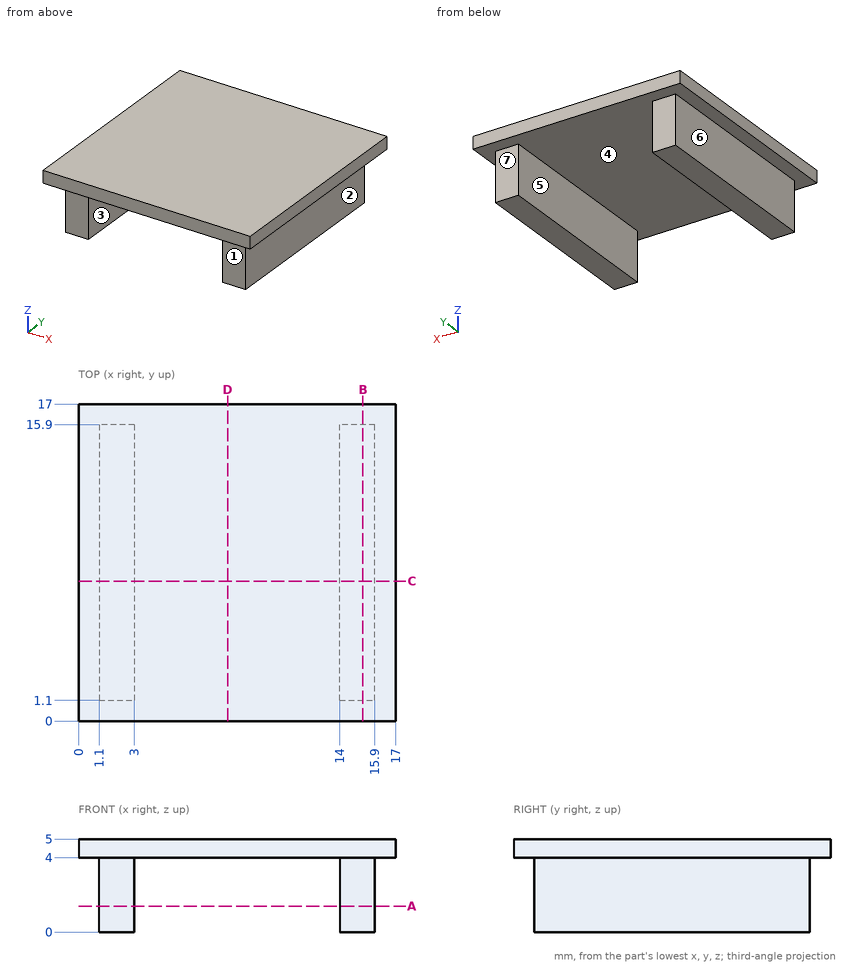
Answer from the drawing. Dimensions are ordinates in mm from the lowest x, y and z of the part. A direction names the side the tool comes from. Round coordinates to 2 decimals unless told otherwise and drop trailing zeros. Loops run counter-clockwise (first coordinate to the right, second up) from the corner with the lowest first, then second, coordinate; pieces in that order, holes last. Notation, with made-up numbers: (-23.5, 28) - (14.5, 28) arc R7 ccw to (14.5, 41) - close; hole circle Ø5 at (9.5, 24). An arc over 180 degrees is marked (long way). Return JSON: item names as keys, results as strings. Group by question number.
1. The part is cut by section A-A on z = 1.4. Determine the outline of the cut face in (x, y), then the cut area to 3 significant figures.
2. Which of the six approach directions +Z, -Z, +X, -X, +Y, -Y give full straight-line access (tool end or side, diameter ignored) to the marked faces 1, 2 and 3?
3. Each of these flat-tipped pins is pushed along its axis until it touches: P1, Ø2, axis at y = 8, z = 1.5, coming from the -X side; P2, Ø2, axis at x = 14.5, z = 2, coming from the -Y side; P3, Ø1, axis at x = 12, z = 3, coming from the +Y side; P4, Ø2, axis at x = 15, z = 1, coming from the +Y side. Where does it stop, or does it pass through?
4. The part is cut by section D-D on x = 8. Determine the outline of the cut face in (y, z).
5. The mould has two halves that part along X. Classify the marked faces 4, 5, 6 and 7: pulls with the +X half, pulls with the -X half, needs draft (parallel to the pull), parting line crosses it, or undercut.
6. Consider probe 1 along X at (y, z) = (7.75, 2.55); probe 2 along Z at (x, y) = (10.5, 14); probe 3 along Y at (x, z) = (14.5, 2.75). Determine where each line is inside the solid, lowest interval first.
7. The part is cut by section B-B on x = 15.25. Determine the outline of the cut face in (y, z).
8. The part is cut by section C-C on y = 7.5. Determine the outline of the cut face in (x, z), then the cut area to 3 significant figures.
Resolved:
{
 "1": {"outline": "(1.1, 1.1) - (3, 1.1) - (3, 15.9) - (1.1, 15.9) - close; (14, 1.1) - (15.9, 1.1) - (15.9, 15.9) - (14, 15.9) - close", "area": "56.2 mm²"},
 "2": {"face 1": "-Z, +X, -X, -Y", "face 2": "-Z, +X, +Y, -Y", "face 3": "-Z, +Y, -Y"},
 "3": {"P1": "stops at x = 1.1", "P2": "stops at y = 1.1", "P3": "passes through", "P4": "stops at y = 15.9"},
 "4": {"outline": "(0, 4) - (17, 4) - (17, 5) - (0, 5) - close"},
 "5": {"face 4": "undercut", "face 5": "undercut", "face 6": "pulls with the -X half", "face 7": "needs draft"},
 "6": {"probe 1": "x = 1.1 to 3, 14 to 15.9", "probe 2": "z = 4 to 5", "probe 3": "y = 1.1 to 15.9"},
 "7": {"outline": "(0, 4) - (1.1, 4) - (1.1, 0) - (15.9, 0) - (15.9, 4) - (17, 4) - (17, 5) - (0, 5) - close"},
 "8": {"outline": "(0, 4) - (1.1, 4) - (1.1, 0) - (3, 0) - (3, 4) - (14, 4) - (14, 0) - (15.9, 0) - (15.9, 4) - (17, 4) - (17, 5) - (0, 5) - close", "area": "32.2 mm²"}
}
